Geometry: final body of the model. Coordinates: model frame, mm. A direction names the side the tool comes from. Give positions to 0.01 mm unless a question says otherwise; leave off trailing zeros. Write each loop counter-clockwise with the first axis right and the second up, starting at its lowest first coordinate (ties: lowest second). Pieces come first, ordered by that corner, then holes.
Q1. Section A-A (z = 39.5). Return the cut outline in (x, y) (3 decimals), plus the area to 3 significant figures.
Q2. Pin query (flat end, axial travel): pin 1 Ø7 at (x, y) = (-40, -24) entering from +Z; pin 2 Ø9.5 at (x, z) = (0, 39.5) entering from -Y; pin 3 Ø3 at (x, z) = (-38, 11) entering from -Y; pin 4 Ø2 at (x, z) = (-17, 40.5) entering from -Y. Return the tip coordinate at first contact, or that it passes through.
Q3. Reachability of faces 5 (the flat face through (1, 26, 46)), 6 (the cylindrical face through (37, -24, 4)) from +Z, -Z, +X, -X, +Y, -Y: full face, straight path, thin tool, end or side. Return the list, or none.
Q4. Line query: line 1 (Y direction, x = 40, z = 2.5); line 2 (Z direction, x = 0, y = 29) (3 decimals); line 3 (X direction, y = 30, z = 39). Output: solid intervals per line, ascending.
Q5. Mould query, pull axis X, two halves, no side actions, for faces 1 (the cylindrical face through (37, 6, 4)), 2 (the flat face through (-50, 28, 19)), 3 (the flat face through (-1, -5, 8)), 4 (the flat face through (50, 28, 19)). Classes: +X half, -X half, draft (parallel to the pull), parting line (faces both ways), or undercut.
Q6. Section B-B (y = -24). Return the cut outline in (x, z), plus the area to 3 significant figures.
Q7. Section C-C (x = -11). Return the cut outline in (y, z).
Q8. Section D-D (z = 29). Return the cut outline in (x, y), plus the area to 3 significant figures.
Autodesk Fusion 360 part; units mm, degrees
sketch "Boceto1" plane through (0, 0, 0) normal (0, 0, 1) x (1, 0, 0)
  line L0 (50, -34) -> (-50, -34)
  line L1 (-50, -34) -> (-50, 34)
  line L2 (-50, 34) -> (50, 34)
  line L3 (50, 34) -> (50, -34)
  line L4 (50, -34) -> (-50, 34) construction
  line L5 (-50, -34) -> (50, 34) construction
  circle A0 centre (-40, 6) radius 3
  circle A1 centre (-40, -24) radius 3
  line L6 (0, -34) -> (0, 34) construction
  circle A2 centre (40, 6) radius 3
  circle A3 centre (40, -24) radius 3
  dimension "d1" = 100
  dimension "d2" = 68
  dimension "d3" = 6
  dimension "d4" = 6
  dimension "d5" = 30
  dimension "d6" = 10
  dimension "d7" = 10
  dimension "d8" = 10
extrude "Extruir1" add sketch "Boceto1" along normal blind 8
sketch "Boceto2" plane through (0, 34, 0) normal (0, 1, 0) x (-1, 0, 0)
  line L0 (-50, 0) -> (50, 0)
  line L1 (50, 0) -> (50, 8)
  line L2 (50, 8) -> (-50, 8)
  line L3 (-50, 8) -> (-50, 0)
  line L4 (-50, 0) -> (-50, 68)
  line L5 (-50, 68) -> (50, 68)
  line L6 (50, 68) -> (50, 0)
  circle A0 centre (0, 39.5) radius 5.175
  dimension "d16" = 68
  dimension "d17" = 10.35
  dimension "d18" = 50
  dimension "d19" = 28.5
extrude "Extruir2" add sketch "Boceto2" against normal blind 8 contours L2 L4 L5 L6
chamfer "Chaflán1" distance 3 angle 45 1 edges at (0, 26, 8)
Computed:
1. outline: (-50, 26) - (-5.175, 26) - (-5.175, 34) - (-50, 34) - close; (5.175, 26) - (50, 26) - (50, 34) - (5.175, 34) - close
1. area: 717 mm2
2. pin 1: stops at z = 8
2. pin 2: passes through
2. pin 3: stops at y = 24.5
2. pin 4: stops at y = 26
3. face 5: +Z, +X, -X, -Y
3. face 6: +Z, -Z
4. line 1: y = -34 to -27, -21 to 3, 9 to 34
4. line 2: z = 0 to 34.325, 44.675 to 68
4. line 3: x = -50 to -5.15, 5.15 to 50
5. face 1: undercut
5. face 2: -X half
5. face 3: draft
5. face 4: +X half
6. outline: (-50, 0) - (-43, 0) - (-43, 8) - (-50, 8) - close; (-37, 0) - (37, 0) - (37, 8) - (-37, 8) - close; (43, 0) - (50, 0) - (50, 8) - (43, 8) - close
6. area: 704 mm2
7. outline: (-34, 0) - (34, 0) - (34, 68) - (26, 68) - (26, 11) - (23, 8) - (-34, 8) - close
8. outline: (-50, 26) - (50, 26) - (50, 34) - (-50, 34) - close
8. area: 800 mm2
